Print and shaded views of the part. All mm, measured from the part's lowest x, y and z. A direction names the side the tool comes from. Give positions to 0.01 mm unless a question says otherwise; leave off trailing zeros. Loops run counter-clockwise (first coordinate to the right, second up) from the corner with the lowest first, then second, coordinate; pieces in that order, holes last. Notation, with made-up numbers: M 68,72 L 89,72 A32 cw 89,101 Z; hole C 18,12.5 d4. An arc over 180 degrees is marked long. Answer in a Markdown table with one row per item.
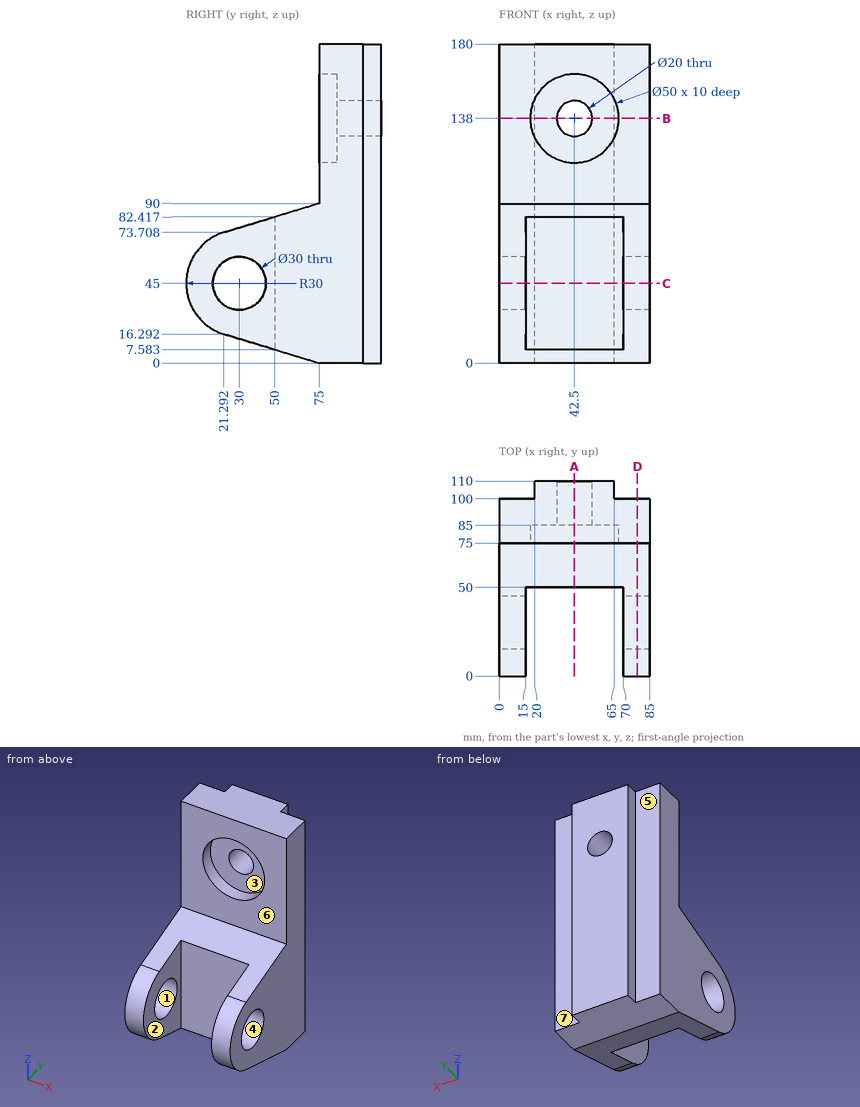
(1) Mould opens along Y. For the marked faces 1, 2, 3 and 4 say: pulls with the +Y half, pulls with the -Y half, needs draft (parallel to the pull), parting line crosses it, or undercut.
Established:
| item | result |
|---|---|
| face 1 | undercut |
| face 2 | needs draft |
| face 3 | pulls with the -Y half |
| face 4 | undercut |
(2) Which spindle directions (+Z, -Z, +X, -X, +Y, -Y) get a long thin tool onto all of the face, cutting with end or side? Do the marked faces 5, 6 and 7. Say none if no direction does.
Established:
| item | result |
|---|---|
| face 5 | +Z, -Z, -X, +Y |
| face 6 | +Z, +X, -X, -Y |
| face 7 | +Z, -Z, +X, +Y |
(3) Saw through at A-A, the plane x = 42.5. Give the cut face in (y, z).
Established:
| item | result |
|---|---|
| outline | M 50,7.58 L 75,0 L 110,0 L 110,128 L 85,128 L 85,113 L 75,113 L 75,90 L 50,82.42 Z; M 75,163 L 85,163 L 85,148 L 110,148 L 110,180 L 75,180 Z |
(4) Wall check: L1, parallel to Z at x = 42.5, y = 96.5; L2, parallel to Z at x = 42.5, y = 81.25; L3, parallel to Y at x = 46, z = 127. Give the ranges that are in metal, low to high.
Established:
| item | result |
|---|---|
| L1 | z = 0 to 128, 148 to 180 |
| L2 | z = 0 to 113, 163 to 180 |
| L3 | y = 85 to 110 |
(5) Saw through at D-D, the plane x = 78. Give the cut face in (y, z).
Established:
| item | result |
|---|---|
| outline | M 21.29,16.29 L 75,0 L 100,0 L 100,180 L 75,180 L 75,90 L 21.29,73.71 A30 ccw Z; hole C 30,45 d30 |
(6) Saw through at B-B, the plane z = 138. Give the cut face in (x, y), and give its area (4 significant figures).
Established:
| item | result |
|---|---|
| outline | M 0,75 L 17.5,75 L 17.5,85 L 32.5,85 L 32.5,110 L 20,110 L 20,100 L 0,100 Z; M 52.5,85 L 67.5,85 L 67.5,75 L 85,75 L 85,100 L 65,100 L 65,110 L 52.5,110 Z |
| area | 1,575 mm2 |
(7) Flat gauge pins, fed straight in: P1, Ø6, axis at x = 13.5, z = 133.5, coming from the +Y side; P2, Ø1, axis at x = 22.5, z = 159, coming from the -Y side; P3, Ø8, axis at x = 73, y = 52, coming from the +Z side. Where does each tip first touch, or does it go through?
Established:
| item | result |
|---|---|
| P1 | stops at y = 100 |
| P2 | stops at y = 75 |
| P3 | stops at z = 84.24 |
(8) Saw through at C-C, the plane z = 45. Give the cut face in (x, y), and give its area (3 significant figures).
Established:
| item | result |
|---|---|
| outline | M 0,0 L 15,0 L 15,15 L 0,15 Z; M 0,45 L 15,45 L 15,50 L 70,50 L 70,45 L 85,45 L 85,100 L 65,100 L 65,110 L 20,110 L 20,100 L 0,100 Z; M 70,0 L 85,0 L 85,15 L 70,15 Z |
| area | 5,300 mm2 |
